Can you work these out from the model? Positions are in its coordinate system, mm. A direction names the side the tool comes from. Give positions to 0.01 mm unless a question says otherwise; leave off trailing zeros. Order: outer loops, then holes, each group sorted by start corner. A loop starts at its lowest first (then second) coordinate and runs counter-clockwise, first axis right, second up. Notation, with made-up numbers: (25.5, 48) - (47.5, 48) arc R24 ccw to (47.5, 60) - close; hole circle Ø3 at (-9.5, -12.75). An arc over 180 degrees is marked (long way). Write each question's results on one line, items separated by ' | '. Start each with the question number.
from build123d import *

# Parameters (mm, degrees)
F1_DEPTH = 63.5
F0_W     = 19.1631158481
F0_H     = 19.05
F2_DEPTH = 25.4
F3_DEPTH = 7.9375
F4_R     = 6.35


with BuildPart() as f1:
    # F0 (on Front) → F1 (new body, symmetric)
    with BuildSketch(Plane.XZ):
        Polygon((22.225, 9.525), (-41.275, 9.525), (-41.275, -9.525), (41.275, -9.525), (41.275, 9.525), align=None)
    extrude(amount=F1_DEPTH, both=True)

    # F0 (on Front) → F2 (join, symmetric)
    with BuildSketch(Plane.XZ):
        with BuildLine():
            Line((22.225, 27.0002), (22.225, 9.525))
            Line((22.225, 9.525), (41.275, 9.525))
            Line((41.275, 9.525), (41.275, 27.0002))
            ThreePointArc((41.275, 27.0002), (45.9246798487, 38.2255201513), (57.15, 42.8752))
            Line((57.15, 42.8752), (60.325, 42.8752))
            Line((60.325, 42.8752), (60.325, 61.9252))
            Line((60.325, 61.9252), (57.15, 61.9252))
            ThreePointArc((57.15, 61.9252), (32.4542956671, 51.6959043329), (22.225, 27.0002))
        make_face()
        with Locations((69.9065579241, 52.4002)):
            Rectangle(F0_W, F0_H)
    extrude(amount=F2_DEPTH, both=True)

    # F0 (on Front) → F3 (join, symmetric)
    with BuildSketch(Plane.XZ):
        with BuildLine():
            add(Edge.make_bspline(
                [(-41.275, 9.525), (-19.9898480937, 42.9106190082), (22.3848360241, 68.1215267785), (57.15, 61.9252)],
                knots=[0, 0, 0, 0, 111.5045361635, 111.5045361635, 111.5045361635, 111.5045361635], degree=3))
            Line((-41.275, 9.525), (22.225, 9.525))
            Line((22.225, 9.525), (22.225, 27.0002))
            ThreePointArc((22.225, 27.0002), (32.4542956671, 51.6959043329), (57.15, 61.9252))
        make_face()
    extrude(amount=F3_DEPTH, both=True)

    # F4
    f4_edges = [f1.edges().sort_by_distance(p)[0] for p in [
        (-41.275, -63.5, 0),
        (41.275, -63.5, 0),
        (41.275, 63.5, 0),
        (-41.275, 63.5, 0),
    ]]
    fillet(f4_edges, radius=F4_R)

    # F0 (on Front) → F5 (revolve)
    with BuildSketch(Plane.XZ):
        Polygon((79.4881158481, 66.675), (79.4881158481, 61.9252), (79.4881158481, 42.8752), (79.4881158481, 38.1), (111.125, 38.1), (111.125, 66.675), align=None)
    revolve(axis=Axis((79.4881158481, 0, 52.3875), (0, 0, 1)))


solid = f1.part
Q1. Thinking about a two-plate mould opening in X: for faces 5 (the flat face through (79, 0, 66.675)), 6 (the cylindrical face through (44.047, -0.356, 35.962)), 7 (the flat face through (41.275, -1, 4)), which applies, released by +X, released by -X, zero draft, split by the parting line, or undercut?
Q2. If we section it at D-D (x = 88): Please give me the cut outline in (y, z) (3 decimals).
Q3. If I drill on probe 1 along Y at (x, z) = (-21.5, 15.5); probe 2 along Z at (x, y) = (77, -20.5) (3 decimals); probe 3 along X at (y, z) = (-20.5, 12.5) (3 decimals), over which ranges is the centre line in solid material (lowest first)? Write a range as from..to.
Q4. If we section it at B-B (y = -10.5): Please give me the cut outline in (x, z) (3 decimals), plus the area to 3 significant figures.
Q5. If we section it at A-A (x = 52): Please give me the cut outline in (y, z) (3 decimals).
Q6. Which directions (+Z, -Z, +X, -X, +Y, -Y) give clear straight access to the entire face, cutting with the end or side of a thin tool? Please do faces 1 (the flat face through (22.225, -17, 18)), 2 (the flat face through (0, -63.5, 0)), 3 (the flat face through (80, 0, 38.1)), 4 (the flat face through (37, 25.4, 36)).
Q7. If we section it at C-C (y = 34): Please give me the cut outline in (x, z) (3 decimals).
Q8. Will these pins go through, and if not, where does the flat tip stop? P1, Ø5, axis at y = -18.5, z = 18, coming from the -X side (3 decimals); P2, Ø8, axis at x = 58, y = -31, coming from the -Z side; P3, Ø5, axis at y = 3, z = 38.5, coming from the -X side; P4, Ø16.5, axis at x = -8.5, y = 46.5, coming from the +Z side (3 decimals).
Findings below:
1) face 5: zero draft | face 6: undercut | face 7: released by +X
2) outline: (-30.47, 38.1) - (30.47, 38.1) - (30.47, 66.675) - (-30.47, 66.675) - close
3) probe 1: y = -7.94..7.94 | probe 2: z = 38.1..66.675 | probe 3: x = 22.225..41.275
4) outline: (-41.275, -9.525) - (41.275, -9.525) - (41.275, 27) arc R15.875 cw to (49.644, 40.989) - (49.644, 38.1) - (109.332, 38.1) - (109.332, 66.675) - (49.644, 66.675) - (49.644, 61.109) arc R34.925 ccw to (22.225, 27) - (22.225, 9.525) - (-41.275, 9.525) - close | area: 4,230 mm2
5) outline: (-25.4, 42.017) - (-15.662, 42.017) - (-15.662, 38.1) - (15.662, 38.1) - (15.662, 42.017) - (25.4, 42.017) - (25.4, 61.543) - (15.662, 61.543) - (15.662, 66.675) - (-15.662, 66.675) - (-15.662, 61.543) - (-25.4, 61.543) - close
6) face 1: +Z, -X, -Y | face 2: +Z, -Z, +X, -X, -Y | face 3: -Z, +X, +Y, -Y | face 4: +Z, -X, +Y
7) outline: (-41.275, -9.525) - (41.275, -9.525) - (41.275, 9.525) - (-41.275, 9.525) - close
8) P1: stops at x = 22.225 | P2: passes through | P3: stops at x = -18.07 | P4: stops at z = 9.525
